from build123d import *

# Parameters (mm, degrees)
SKETCH1_W           = 20.576108637
SKETCH1_H           = 33.628117847
SKETCH1_R           = 5.1
SKETCH1_R_2         = 1.6
BOSS_EXTRUDE1_DEPTH = 18.9
SKETCH3_W           = 12
SKETCH3_H           = 18.9
BOSS_EXTRUDE3_DEPTH = 11
SKETCH4_R           = 1.9
BOSS_EXTRUDE6_DEPTH = 2
BOSS_EXTRUDE7_START = 2
SKETCH5_R           = 1.9
BOSS_EXTRUDE7_DEPTH = 2
CUT_EXTRUDE1_DEPTH  = 40.488623232
CUT_EXTRUDE2_DEPTH  = 40.488623232
SKETCH8_W           = 10.181570082
SKETCH8_H           = 10.9
CUT_EXTRUDE3_DEPTH  = 6
SKETCH9_R           = 6.144425542
BOSS_EXTRUDE8_DEPTH = 10
SKETCH10_R          = 3
CUT_EXTRUDE4_DEPTH  = 6


with BuildPart() as part:
    # Sketch1 → Boss-Extrude1 (new body)
    with BuildSketch(Plane.XY):
        with Locations((9.059629922, -0.460659149)):
            Rectangle(SKETCH1_W, SKETCH1_H)
        with Locations((8.525263921, 7.417965689)):
            Circle(SKETCH1_R, mode=Mode.SUBTRACT)
        with Locations((3.37816709, -9.67384212)):
            Circle(SKETCH1_R_2, mode=Mode.SUBTRACT)
    extrude(amount=BOSS_EXTRUDE1_DEPTH)

    # Sketch3 → Boss-Extrude3 (add)
    with BuildSketch(Plane(origin=(0, 16.353399775, 0), x_dir=(1, 0, 0), z_dir=(0, 1, 0))):
        with Locations((4.771575604, -9.45)):
            Rectangle(SKETCH3_W, SKETCH3_H)
    extrude(amount=BOSS_EXTRUDE3_DEPTH)

    # Sketch4 → Boss-Extrude6 (add)
    with BuildSketch(Plane.XY.offset(18.9)):
        with Locations((1.771575604, 24.353399775)):
            Circle(SKETCH4_R)
    extrude(amount=BOSS_EXTRUDE6_DEPTH)

    # Sketch5 → Boss-Extrude7 (add)
    with BuildSketch(Plane(origin=(0, 0, 0), x_dir=(-1, 0, 0), z_dir=(0, 0, -1)).offset(BOSS_EXTRUDE7_START)):
        with Locations(Location((-1.771575604, 24.353399775, 0), (0, 0, 180))):
            Circle(SKETCH5_R)
    extrude(amount=-BOSS_EXTRUDE7_DEPTH)

    # Sketch6 → Cut-Extrude1 (cut, through all)
    with BuildSketch(Plane.XY.offset(18.9)):
        Polygon((5.606824739, -17.274718072), (19.347684241, 4.666075764), (19.347684241, -17.274718072), align=None)
    extrude(amount=-CUT_EXTRUDE1_DEPTH, mode=Mode.SUBTRACT)

    # Sketch7 → Cut-Extrude2 (cut, through all)
    with BuildSketch(Plane.XY.offset(18.9)):
        Polygon((5.334321987, 27.353399775), (10.771575604, 19.908581769), (10.771575604, 27.353399775), align=None)
    extrude(amount=-CUT_EXTRUDE2_DEPTH, mode=Mode.SUBTRACT)

    # Sketch8 → Cut-Extrude3 (cut)
    with BuildSketch(Plane(origin=(0, 27.353399775, 0), x_dir=(1, 0, 0), z_dir=(0, 1, 0))):
        with Locations((3.862360645, -9.45)):
            Rectangle(SKETCH8_W, SKETCH8_H)
    extrude(amount=-CUT_EXTRUDE3_DEPTH, mode=Mode.SUBTRACT)

    # Sketch9 → Boss-Extrude8 (add)
    with BuildSketch(Plane.XY.offset(18.9)):
        with Locations((8.525263921, 7.417965689)):
            Circle(SKETCH9_R)
    extrude(amount=-BOSS_EXTRUDE8_DEPTH)

    # Sketch10 → Cut-Extrude4 (cut)
    with BuildSketch(Plane.XY.offset(18.9)):
        with Locations((3.37816709, -9.67384212)):
            Circle(SKETCH10_R)
    extrude(amount=-CUT_EXTRUDE4_DEPTH, mode=Mode.SUBTRACT)


solid = part.part
Can you work these out from the model? Positions are in its coordinate system, mm. A direction names the side the tool comes from. Coordinates: 2 decimals unless noted, no trailing zeros. Loops run counter-clockwise (first coordinate to the right, second up) from the corner with the lowest first, then second, coordinate; pieces in that order, holes last. Notation, with made-up numbers: M -1.75,85.5 L 36.25,85.5 A22 cw 36.25,119.5 Z; hole C 11.25,-17.5 d3. An arc over 180 degrees is marked long. Return JSON: item names as keys, results as strings. Group by question number.
Item 1: I'm going to push flat-ended pins straight in: pin 1 Ø8 at (x, z) = (15.5, 10) entering from -Y; pin 2 Ø2 at (x, y) = (1.5, -4.5) entering from +Z; pin 3 Ø3 at (y, z) = (19, 9.5) entering from +X; pin 4 Ø2.5 at (x, y) = (3.38, -9.67) entering from -Z. Where does each tip first touch, or does it pass through?
Item 2: Thinking about a two-plate mould opening in X: for faces 5 (the flat face through (2, 27.353, 17)), 6 (the cylindrical face through (3.43, 7.64, 4.39)), 7 (the flat face through (10.772, 18, 10)), 8 (the flat face through (8.953, 22, 10)), which applies, released by +X, released by -X, zero draft, split by the parting line, or undercut?
Item 3: If I drill on L1, parallel to Z at x = 0.75, y = 22.5; L2, parallel to Z at x = 1.5, y = 24; L3, parallel to Z at x = 8.5, y = 16, over which ranges is the centre line in solid material (lowest first)? Write a range as from..to.
Item 4: Imagine slicing it at B-B (x = 12.25). Please give me the cut outline in (y, z).
Item 5: Imagine slicing it at D-D (y = 12). Please give me the cut outline in (x, z).
Item 6: Imagine slicing it at C-C (z = 17.5). Please give me the cut outline in (x, y).
Item 7: On a 3-axis mill with a long thin cutter (end or side, diameter ignored), from which of +Z, -Z, +X, -X, +Y, -Y can I reach the whole of each face in a straight line? I mean faces 1 (the flat face through (15, 16.353, 9)), 2 (the flat face through (5, -11, 12.9)), 3 (the flat face through (3, 24, 14.9)), 4 (the flat face through (8, 7, 8.9)). Say none if no direction works.
Item 8: Imagine slicing it at A-A (z = 5.5). Please give me the cut outline in (x, y), and give its area (3 significant figures).
Verdict:
{
 "1": {"pin 1": "stops at y = -7.86", "pin 2": "stops at z = 18.9", "pin 3": "stops at x = 10.77", "pin 4": "passes through"},
 "2": {"face 5": "zero draft", "face 6": "undercut", "face 7": "released by +X", "face 8": "released by -X"},
 "3": {"L1": "z = 0..4, 14.9..18.9", "L2": "z = -2..4, 14.9..20.9", "L3": "z = 0..18.9"},
 "4": {"outline": "M -6.67,0 L 3.93,0 L 3.93,8.9 L 10.9,8.9 L 10.9,0 L 16.35,0 L 16.35,18.9 L -6.67,18.9 Z"},
 "5": {"outline": "M -1.23,0 L 6.29,0 L 6.29,8.9 L 10.76,8.9 L 10.76,0 L 19.35,0 L 19.35,18.9 L -1.23,18.9 Z"},
 "6": {"outline": "M -1.23,-17.27 L 5.61,-17.27 L 19.35,4.67 L 19.35,16.35 L 10.77,16.35 L 10.77,19.91 L 5.33,27.35 L -1.23,27.35 Z; hole C 3.38,-9.67 d6"},
 "7": {"face 1": "+Z, -Z, +X, +Y", "face 2": "+Z", "face 3": "-X, +Y", "face 4": "-Z"},
 "8": {"outline": "M -1.23,-17.27 L 5.61,-17.27 L 19.35,4.67 L 19.35,16.35 L 10.77,16.35 L 10.77,19.91 L 8.95,22.4 L 8.95,21.35 L -1.23,21.35 Z; hole C 3.38,-9.67 d3.2; hole C 8.53,7.42 d10.2", "area": "511 mm^2"}
}
